from build123d import *

# Parameters (mm, degrees)
CROQUIS1_W              = 90
CROQUIS1_H              = 47
SALIENTE_EXTRUIR1_DEPTH = 3
CROQUIS2_W              = 90
CROQUIS2_H              = 47
CROQUIS2_W_2            = 84
CROQUIS2_H_2            = 41
SALIENTE_EXTRUIR2_DEPTH = 40
CROQUIS6_W              = 72
CROQUIS6_H              = 25
CORTAR_EXTRUIR5_DEPTH   = 3
CROQUIS8_W              = 34
CROQUIS8_H              = 15
CORTAR_EXTRUIR6_DEPTH   = 3
CROQUIS9_W              = 9.999999999
CROQUIS9_H              = 5
SALIENTE_EXTRUIR3_DEPTH = 7
CROQUIS10_W             = 3
CROQUIS10_H             = 20
SALIENTE_EXTRUIR4_DEPTH = 20
CROQUIS12_W             = 3
CROQUIS12_H             = 20
SALIENTE_EXTRUIR5_DEPTH = 20
CROQUIS13_W             = 10
CROQUIS13_H             = 5
SALIENTE_EXTRUIR6_DEPTH = 7
CROQUIS14_W             = 11
CROQUIS14_H             = 6
CORTAR_EXTRUIR8_DEPTH   = 3
CROQUIS15_R             = 9
CROQUIS15_W             = 7
CROQUIS15_H             = 5
CROQUIS15_W_2           = 6
CROQUIS15_H_2           = 8
CORTAR_EXTRUIR9_DEPTH   = 3


with BuildPart() as part:
    # Croquis1 → Saliente-Extruir1 (new body)
    with BuildSketch(Plane(origin=(0, 0, 0), x_dir=(1, 0, 0), z_dir=(0, 1, 0))):
        Rectangle(CROQUIS1_W, CROQUIS1_H)
    extrude(amount=SALIENTE_EXTRUIR1_DEPTH)

    # Croquis2 → Saliente-Extruir2 (add)
    with BuildSketch(Plane(origin=(0, 3, 0), x_dir=(1, 0, 0), z_dir=(0, 1, 0))):
        Rectangle(CROQUIS2_W, CROQUIS2_H)
        Rectangle(CROQUIS2_W_2, CROQUIS2_H_2, mode=Mode.SUBTRACT)
    extrude(amount=SALIENTE_EXTRUIR2_DEPTH)

    # Croquis6 → Cortar-Extruir5 (cut)
    with BuildSketch(Plane(origin=(0, 0, 0), x_dir=(-1, 0, 0), z_dir=(0, -1, 0))):
        with Locations((0.009067855, 0.029457722)):
            Rectangle(CROQUIS6_W, CROQUIS6_H)
    extrude(amount=-CORTAR_EXTRUIR5_DEPTH, mode=Mode.SUBTRACT)

    # Croquis8 → Cortar-Extruir6 (cut)
    with BuildSketch(Plane(origin=(45, 0, 0), x_dir=(0, 0, -1), z_dir=(1, 0, 0))):
        with Locations((1.598714356, 27.442281593)):
            Rectangle(CROQUIS8_W, CROQUIS8_H)
    extrude(amount=-CORTAR_EXTRUIR6_DEPTH, mode=Mode.SUBTRACT)

    # Croquis9 → Saliente-Extruir3 (add)
    with BuildSketch(Plane(origin=(45, 0, 0), x_dir=(0, 0, -1), z_dir=(1, 0, 0))):
        with Locations((-0.008616077, 40.502224836)):
            Rectangle(CROQUIS9_W, CROQUIS9_H)
    extrude(amount=SALIENTE_EXTRUIR3_DEPTH)

    # Croquis10 → Saliente-Extruir4 (add)
    with BuildSketch(Plane(origin=(45, 0, 0), x_dir=(0, 0, -1), z_dir=(1, 0, 0))):
        with Locations((22.028285353, 21.493620383)):
            Rectangle(CROQUIS10_W, CROQUIS10_H)
    extrude(amount=SALIENTE_EXTRUIR4_DEPTH)

    # Croquis12 → Saliente-Extruir5 (add)
    with BuildSketch(Plane.ZY.offset(45)):
        with Locations((-22.029401758, 21.485642244)):
            Rectangle(CROQUIS12_W, CROQUIS12_H)
    extrude(amount=SALIENTE_EXTRUIR5_DEPTH)

    # Croquis13 → Saliente-Extruir6 (add)
    with BuildSketch(Plane.ZY.offset(45)):
        with Locations((0.007263923, 40.528739096)):
            Rectangle(CROQUIS13_W, CROQUIS13_H)
    extrude(amount=SALIENTE_EXTRUIR6_DEPTH)

    # Croquis14 → Cortar-Extruir8 (cut)
    with BuildSketch(Plane.ZY.offset(45)):
        with Locations((-5.001075708, 18.007541224)):
            Rectangle(CROQUIS14_W, CROQUIS14_H)
    extrude(amount=-CORTAR_EXTRUIR8_DEPTH, mode=Mode.SUBTRACT)

    # Croquis15 → Cortar-Extruir9 (cut)
    with BuildSketch(Plane(origin=(0, 0, -23.5), x_dir=(-1, 0, 0), z_dir=(0, 0, -1))):
        with Locations((-5.958347551, 31.946109842)):
            Circle(CROQUIS15_R)
        with Locations((21.041652448, 31.946109842)):
            Circle(CROQUIS15_R)
        with Locations((33.5380591, 23.898149155)):
            Rectangle(CROQUIS15_W, CROQUIS15_H)
        with Locations((7.510757726, 26.075310147)):
            Rectangle(CROQUIS15_W_2, CROQUIS15_H_2)
    extrude(amount=-CORTAR_EXTRUIR9_DEPTH, mode=Mode.SUBTRACT)


solid = part.part
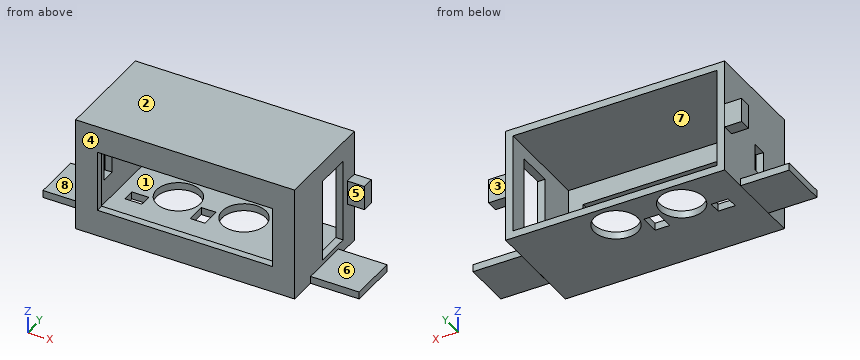
For this review, take the finished solid that the model builds, in its own axes (mm). Face numbers are marked on the shaded views. A direction names the side the tool comes from. Give positions to 0.01 mm unless a question says otherwise; leave off trailing zeros. Order: outer loops, then holes, each group sorted by start corner. A loop starts at its lowest first (then second) coordinate and runs counter-clockwise, first axis right, second up. Notation, with made-up numbers: (-22.5, -34.75) - (-16.5, -34.75) arc R25 cw to (-16.5, -6.75) - close; hole circle Ø3 at (18.25, 5.25). An arc over 180 degrees is marked (long way). Answer as a JSON object with one key per item and string values. Group by question number.
Item 1: Machinability: for the marked faces 4, 5, 6, 7 and 8, which of the approach directions +Z, -Z, +X, -X, +Y, -Y give a long, thin tool a straight path to every point of the face, cutting with its end or side? Answer none if there is none.
Item 2: Take a section at B-B on x = -34.5. Give the boundary of the cut face in (y, z).
Item 3: Clearance check with flat-ended pins moving along their axes: pin 1 Ø6 at (y, z) = (12, 8) entering from +X; pin 2 Ø23.5 at (x, y) = (-21.04, 31.95) entering from -Z; pin 3 Ø1.5 at (y, z) = (41.5, -0.5) entering from -X. State where each tip first meets the part, or that it passes through.
Item 4: Draft analysis for pull direction Z (two halves, no side actions). For the marked faces 1, 2 and 3, state which applies: pulls with the +Z half, pulls with the -Z half, needs draft (parallel to the pull), parting line crosses it, or undercut.
Item 5: Take a section at D-D on y = 39.5. Give the boundary of the cut face in (x, z).
Item 6: Wall thickness on line 1 along X through (y, z) = (5, 13); line 2 along Z through (x, y) = (17.5, 15.5); line 3 along X through (y, z) = (27, -9): over which ranges is each line inside the solid? List them lowest first.
Item 7: Take a section at A-A on z = -1. Give the number of separate pieces and of enclosed holes in the cut face, and give its area (3 significant figures).
Item 8: Take a section at C-C on x = 43.5. Give the boundary of the cut face in (y, z).
Reported:
{
 "1": {"face 4": "+Z, -Z, +X, -X, -Y", "face 5": "+Z, -Z, +X, -Y", "face 6": "+Z, +X, +Y, -Y", "face 7": "+Y", "face 8": "+Z, -X, +Y, -Y"},
 "2": {"outline": "(0, -23.5) - (21.4, -23.5) - (21.4, -20.5) - (3, -20.5) - (3, -12.53) - (0, -12.53) - close; (0, 12.47) - (3, 12.47) - (3, 20.5) - (43, 20.5) - (43, 23.5) - (0, 23.5) - close; (26.4, -23.5) - (43, -23.5) - (43, -20.5) - (26.4, -20.5) - close"},
 "3": {"pin 1": "x = 45", "pin 2": "z = -23.5", "pin 3": "x = -52"},
 "4": {"face 1": "undercut", "face 2": "pulls with the +Z half", "face 3": "needs draft"},
 "5": {"outline": "(-52, -4.99) - (-45, -4.99) - (-45, -23.5) - (-25.93, -23.5) - (-25.93, -20.5) - (-42, -20.5) - (-42, 20.5) - (42, 20.5) - (42, -20.5) - (10.85, -20.5) - (10.85, -23.5) - (45, -23.5) - (45, -4.99) - (52, -4.99) - (52, 5.01) - (45, 5.01) - (45, 23.5) - (-45, 23.5) - (-45, 5.01) - (-52, 5.01) - close; (-16.15, -23.5) - (1.07, -23.5) - (1.07, -20.5) - (-16.15, -20.5) - close"},
 "6": {"line 1": "-45 to -42, 42 to 45", "line 2": "-23.5 to -20.5, 20.5 to 23.5", "line 3": "-45 to -42"},
 "7": {"separate pieces": "4", "enclosed holes": "0", "area": "301 mm^2"},
 "8": {"outline": "(0, -23.5) - (43, -23.5) - (43, 23.5) - (0, 23.5) - close; hole (19.94, -18.6) - (34.94, -18.6) - (34.94, 15.4) - (19.94, 15.4) - close"}
}
